Input: part model. Units: mm. Frame: model coordinates. Face numbers are marked on the shaded views. Give positions to 0.01 mm unless a question says otherwise; leave off trailing zeros. Write each loop counter-clockwise with the first axis right and the second up, starting at its lowest first coordinate (ties: lowest second). Pieces come first, ordered by that corner, then holes. Notation, with made-up numbers: M 28.25,-33 L 33.25,-33 A30 cw 33.25,4 Z; hole C 80,86.5 d6. An arc over 180 degrees is marked long. Use CSV: the item, a comma, the result in double quotes. Start each with the question number.
from build123d import *

# Parameters (mm, degrees)
SKETCH_W    = 100
SKETCH_H    = 100
SKETCH_R    = 10
PAD_DEPTH   = 10
SKETCH002_R = 1


with BuildPart() as part:
    # Sketch → Pad (new body)
    with BuildSketch(Plane.XY):
        with Locations((50, 50)):
            Rectangle(SKETCH_W, SKETCH_H)
        with Locations((60, 40)):
            Circle(SKETCH_R, mode=Mode.SUBTRACT)
    extrude(amount=PAD_DEPTH)

    # SubtractivePipe: sweep along a path in Sketch001
    with BuildLine(Plane.XY.offset(5)) as subtractivepipe_path:
        Line((-10, 20), (60, 20))
        ThreePointArc((60, 20), (74.142136, 25.857864), (80, 40))
        Line((80, 40), (80, 110))
    # Sketch002 → SubtractivePipe (sweep, cut)
    with BuildSketch(Plane(origin=(0, 0, 5), x_dir=(0, 1, 0), z_dir=(1, 0, 0))):
        with Locations((20, 0)):
            Circle(SKETCH002_R)
    sweep(path=subtractivepipe_path.line, mode=Mode.SUBTRACT)

    # AdditivePipe: sweep along a path in Sketch005
    with BuildLine(Plane.XY.offset(5)) as additivepipe_path:
        Line((0, 20), (60, 20))
        ThreePointArc((60, 20), (74.142136, 25.857864), (80, 40))
        Line((80, 40), (80, 100))
    # Sketch006 → AdditivePipe (sweep)
    with BuildSketch(Plane(origin=(0, 20, 5), x_dir=(0, 1, 0), z_dir=(1, 0, 0))):
        with BuildLine():
            ThreePointArc((0, -1), (0.707107, -0.707107), (1, 0))
            Line((1, 0), (0, 0))
            Line((0, 0), (0, -1))
        make_face()
    sweep(path=additivepipe_path.line)

    # AdditivePipe001: sweep along a path in Sketch011
    with BuildLine(Plane.XY.offset(5)) as additivepipe001_path:
        Line((0, 20), (60, 20))
        ThreePointArc((60, 20), (74.142136, 25.857864), (80, 40))
        Line((80, 40), (80, 100))
    # Sketch012 → AdditivePipe001 (sweep)
    with BuildSketch(Plane(origin=(0, 20, 5), x_dir=(0, 0, 1), z_dir=(1, 0, 0))):
        with BuildLine():
            ThreePointArc((0, -1), (0.707107, -0.707107), (1, 0))
            Line((1, 0), (0, 0))
            Line((0, 0), (0, -1))
        make_face()
    sweep(path=additivepipe001_path.line)

    # AdditivePipe002: sweep along a path in Sketch016
    with BuildLine(Plane.XY.offset(5)) as additivepipe002_path:
        Line((0, 20), (60, 20))
        ThreePointArc((60, 20), (74.142136, 25.857864), (80, 40))
        Line((80, 40), (80, 100))
    # Sketch015 → AdditivePipe002 (sweep)
    with BuildSketch(Plane(origin=(0, 20, 5), x_dir=(0, 0, -1), z_dir=(1, 0, 0))):
        with BuildLine():
            ThreePointArc((0, -1), (0.707107, -0.707107), (1, 0))
            Line((1, 0), (0, 0))
            Line((0, 0), (0, -1))
        make_face()
    sweep(path=additivepipe002_path.line)

    # AdditivePipe003: sweep along a path in Sketch013
    with BuildLine(Plane.XY.offset(5)) as additivepipe003_path:
        Line((0, 20), (60, 20))
        ThreePointArc((60, 20), (74.142136, 25.857864), (80, 40))
        Line((80, 40), (80, 100))
    # Sketch014 → AdditivePipe003 (sweep)
    with BuildSketch(Plane(origin=(0, 20, 5), x_dir=(0, -1, 0), z_dir=(1, 0, 0))):
        with BuildLine():
            ThreePointArc((0, -1), (0.707107, -0.707107), (1, 0))
            Line((1, 0), (0, 0))
            Line((0, 0), (0, -1))
        make_face()
    sweep(path=additivepipe003_path.line)


solid = part.part
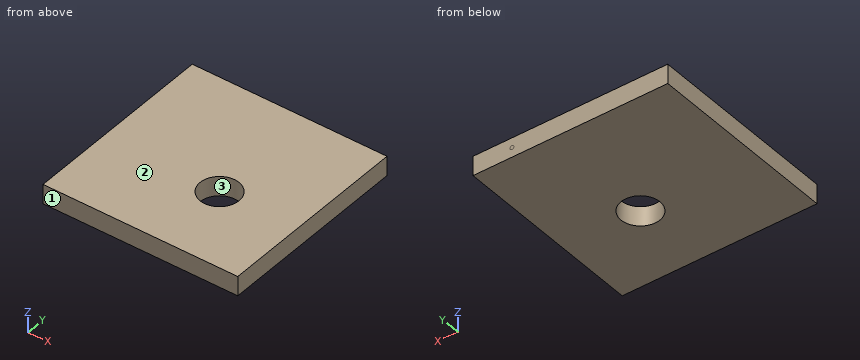
Q1. Section C-C, the plane y = 40. Return the cut outline in (x, z).
Q2. Section B-B, the plane z = 7.5. Return the cut outline in (x, y), and give its area (3 significant figures).
Q3. Pull-direction query (Y, two-part tool) for the marked faces 1, 2 and 3; classes: released by +Y, released by -Y, zero draft, split by the parting line, or undercut.
Q4. First-contact query: pin 1 Ø12 at (x, y) = (60, 40) entering from -Z. Flat tip, straight axial feed; report the tip coordinate or a pass-through.
Q5. Material intervals for L1, parallel to Y at x = 60, z = 5.5; L2, parallel to Y at x = 67.5, z = 4; L3, parallel to X at y = 32.5, z = 6.75, sorted ascending. Write a range as [from, to].
Q6. Section A-A, the plane x = 60. Return the cut outline in (y, z), and give its area (3 significant figures).
Check result:
1,outline,"M 0,0 L 50,0 L 50,10 L 0,10 Z; M 70,0 L 100,0 L 100,10 L 70,10 Z"
2,outline,"M 0,0 L 100,0 L 100,100 L 0,100 Z; hole C 60,40 d20"
2,area,"9,690 mm²"
3,face 1,"released by -Y"
3,face 2,"zero draft"
3,face 3,"undercut"
4,pin 1,"passes through"
5,L1,"y = [0, 30], [50, 100]"
5,L2,"y = [0, 33.39], [46.61, 100]"
5,L3,"x = [0, 53.39], [66.61, 100]"
6,outline,"M 0,0 L 30,0 L 30,10 L 0,10 Z; M 50,0 L 100,0 L 100,10 L 50,10 Z"
6,area,"800 mm²"
